Work out the finished part from the listing and answer in its coordinate system (mm). Face numbers are marked on the shaded views. Round coordinates to 2 decimals unless told otherwise and drop trailing zeros. Loops run counter-clockwise (first coordinate to the right, second up) from the corner with the lowest first, then second, coordinate; pieces in that order, holes last.
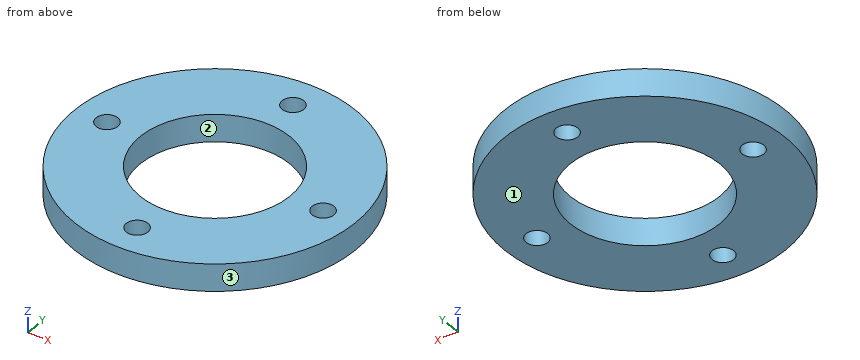
Autodesk Inventor part; units mm, degrees
ref_plane "YZ Plane" through (0, 0, 0) normal (1, 0, 0) x (0, 1, 0)
ref_plane "XZ Plane" through (0, 0, 0) normal (0, 1, 0) x (-1, 0, 0)
ref_plane "XY Plane" through (0, 0, 0) normal (0, 0, 1) x (1, 0, 0)
sketch "Sketch1" plane through (0, 0, 0) normal (0, 0, 1) x (1, 0, 0)
  circle A0 centre (0, 0) radius 11
  circle A1 centre (0, 0) radius 20.6625
  point P0 (16, 0)
  point P1 (0, 16)
  point P2 (-16, 0)
  point P3 (0, -16)
  dimension "d0" = 22
  dimension "d2" = 16
  dimension "d5" = 360
  dimension "d7" = 41.325
extrude "Plate1" add sketch "Sketch1" along normal blind 4
hole "Hole1" at (16, 0, 0) at (0, 16, 0) at (-16, 0, 0) at (0, -16, 0) direction (0, 0, 1) diameter 3.2 end through all
equation "\"d14\" = Thickness"
equation "\"d8\" = Thickness"
equation "\"BendRadius\" = Thickness"
equation "\"BendReliefWidth\" = Thickness"
equation "\"BendReliefDepth\" = 0.5 * Thickness"
equation "\"CornerReliefSize\" = 4 * Thickness"
equation "\"MinimumRemnant\" = 2 * Thickness"
equation "\"TransitionRadius\" = BendRadius"
equation "\"JacobiRadiusSize\" = BendRadius"
equation "\"GapSize\" = Thickness"
properties part number "spacer 4 mm" material "Aluminum 6061"
1. Determine the mould class of the marked faces 1, 2 and 3 for opening direction X: +X half, -X half, draft (parallel to the pull), parting line (faces both ways), or undercut.
Answer key:
face 1: draft
face 2: undercut
face 3: parting line
2. Find section C-C (y = 7). Write down the section's boundary in (x, z).
Answer key:
outline: (-19.44, 0) - (-8.49, 0) - (-8.49, 4) - (-19.44, 4) - close; (8.49, 0) - (19.44, 0) - (19.44, 4) - (8.49, 4) - close
3. Find section A-A (y = 0). Write down the section's boundary in (x, z).
Answer key:
outline: (-20.66, 0) - (-17.6, 0) - (-17.6, 4) - (-20.66, 4) - close; (-14.4, 0) - (-11, 0) - (-11, 4) - (-14.4, 4) - close; (11, 0) - (14.4, 0) - (14.4, 4) - (11, 4) - close; (17.6, 0) - (20.66, 0) - (20.66, 4) - (17.6, 4) - close
4. Find section B-B (x = -16). Write down the section's boundary in (y, z).
Answer key:
outline: (-13.07, 0) - (-1.6, 0) - (-1.6, 4) - (-13.07, 4) - close; (1.6, 0) - (13.07, 0) - (13.07, 4) - (1.6, 4) - close
5. Consider probe 1 along Y at (x, z) = (0, 0.9); probe 2 along X at (y, z) = (-1, 2.9); probe 3 along X at (y, z) = (-5, 1.25). Determine where each line is inside the solid, lowest interval first.
Answer key:
probe 1: y = -20.66 to -17.6, -14.4 to -11, 11 to 14.4, 17.6 to 20.66
probe 2: x = -20.64 to -17.25, -14.75 to -10.95, 10.95 to 14.75, 17.25 to 20.64
probe 3: x = -20.05 to -9.8, 9.8 to 20.05
6. Given pin 1 (2 mm diameter, centred on x = -7.5, z = 0.5, fed in from -Y); pin 2 (5 mm diameter, centred on x = -16, y = 0, fed in from -Z); pin 3 (1 mm diameter, centred on y = -3.5, z = 3, fed in from +X); pin 4 (1 mm diameter, centred on y = 12.5, z = 2, fed in from -X), each flat-ended and moving along its own axis, determine where each tip first touches the part or whether it passes through.
Answer key:
pin 1: stops at y = -19.61
pin 2: stops at z = 0
pin 3: stops at x = 20.44
pin 4: stops at x = -16.82
7. Find section D-D (z = 1.5). Write down the section's boundary in (x, y) (1 decimal).
Answer key:
outline: circle Ø41.3 at (0, 0); hole circle Ø3.2 at (-16, 0); hole circle Ø22 at (0, 0); hole circle Ø3.2 at (0, -16); hole circle Ø3.2 at (0, 16); hole circle Ø3.2 at (16, 0)
